The model under review builds one solid part; all positions refer to its coordinate system, in mm. A direction names the side the tool comes from. Round coordinates to 2 decimals unless told otherwise and drop trailing zeros. Write each loop counter-clockwise with the first axis right and the second up, starting at its lowest first coordinate (ties: lowest second). Pieces come first, ordered by that corner, then holes. Notation, with made-up numbers: (38, 14) -> (48, 14) arc R20 cw to (48, 43) -> close; hole circle Ø6 at (-17.75, 60.25). An arc over 180 degrees is marked (long way). Use CSV: the item, a comma, the result in double quotes. Start each with the question number.
1) Wall thickness on probe 1 along Y at (x, z) = (-0.4, 19.5); probe 2 along X at (y, z) = (-0.75, 12); probe 3 along Y at (x, z) = (10, 21): over which ranges is each line inside the solid? List them lowest first. Write a range as [from, to].
2) Machinability: for faces 4 (the face through (1, -7, 20)), 5 (the face through (4.5, 0, 20)), 6 (the face through (10.768, 7.436, 20.88)), which of the approach directions +Z, -Z, +X, -X, +Y, -Y give a long, thin tool a straight path to every point of the face, cutting with its end or side? Answer none if there is none.
3) Take a section at A-A, the plane x = -9.5. Give the boundary of the cut face in (y, z), then the cut area to 3 significant figures.
4) For pin 1 Ø6 at (y, z) = (-4, 5) entering from +X; pin 2 Ø7 at (y, z) = (5, 19.5) entering from +X; pin 3 Ø3 at (y, z) = (-4, 19.5) entering from +X; pin 4 Ø1.2 at (x, y) = (11, 4.5) entering from +Z, all flat-tipped, find the tip position at first contact; note any pin that passes through.
5) Take a section at B-B, the plane z = 12. Give the boundary of the cut face in (x, y), then the cut area to 3 significant figures.
6) Mouldability with a two-part tool opening along Z and no side actions: class faces 1 (the face through (14, 0, 3)), 2 (the face through (10.768, -7.436, 18.12)), 3 (the face through (-16.14, 9.1, 1.52)) as released by +Z, released by -Z, zero draft, split by the parting line, or undercut.
7) Take a section at C-C, the plane y = 0. Give the boundary of the cut face in (x, z), then the cut area to 3 significant figures.
8) Take a section at D-D, the plane y = 4. Give the boundary of the cut face in (x, z).
from build123d import *

# Parameters (mm, degrees)
SKETCH1_W           = 34
SKETCH1_H           = 20
BOSS_EXTRUDE1_DEPTH = 3
FILLET1_R           = 3
SKETCH2_W           = 14
SKETCH2_H           = 20
BOSS_EXTRUDE2_DEPTH = 20
CUT_EXTRUDE1_DEPTH  = 35.899856733
CHAMFER1_SIZE       = 1
SKETCH4_R           = 2.2
CUT_EXTRUDE2_DEPTH  = 29.08914381
SKETCH5_R           = 1.7
CUT_EXTRUDE3_DEPTH  = 39.340579025
FILLET2_R           = 2
CUT_EXTRUDE4_DEPTH  = 2.5
SKETCH7_R           = 2.75
CUT_EXTRUDE5_DEPTH  = 3


with BuildPart() as part:
    # Sketch1 → Boss-Extrude1 (new body)
    with BuildSketch(Plane.XY):
        Rectangle(SKETCH1_W, SKETCH1_H)
    extrude(amount=BOSS_EXTRUDE1_DEPTH)

    # Fillet1
    fillet1_edges = [part.edges().sort_by_distance(p)[0] for p in [
        (17, -10, 1.5),
        (-17, -10, 1.5),
        (-17, 10, 1.5),
        (17, 10, 1.5),
    ]]
    fillet(fillet1_edges, radius=FILLET1_R)

    # Sketch2 → Boss-Extrude2 (add)
    with BuildSketch(Plane.XY.offset(3)):
        with Locations((5, 0)):
            Rectangle(SKETCH2_W, SKETCH2_H)
    extrude(amount=BOSS_EXTRUDE2_DEPTH)

    # Sketch3 → Cut-Extrude1 (cut, through all)
    with BuildSketch(Plane(origin=(0, 10, 0), x_dir=(1, 0, 0), z_dir=(0, 1, 0))):
        with BuildLine():
            Line((4.5, -16.119769411), (4.5, -23))
            Line((4.5, -23), (5.5, -23))
            Line((5.5, -23), (5.5, -16.119769411))
            ThreePointArc((5.5, -16.119769411), (5, -7.85), (4.5, -16.119769411))
        make_face()
    extrude(amount=-CUT_EXTRUDE1_DEPTH, mode=Mode.SUBTRACT)

    # Chamfer1
    chamfer1_edges = [part.edges().sort_by_distance(p)[0] for p in [
        (5, -10, 7.85),
        (5, 10, 7.85),
    ]]
    chamfer(chamfer1_edges, length=CHAMFER1_SIZE)

    # Sketch4 → Cut-Extrude2 (cut, through all)
    with BuildSketch(Plane.XY.offset(3)):
        with Locations((-9.5, 0)):
            Circle(SKETCH4_R)
    extrude(amount=-CUT_EXTRUDE2_DEPTH, mode=Mode.SUBTRACT)

    # Sketch5 → Cut-Extrude3 (cut, through all)
    with BuildSketch(Plane(origin=(12, 0, 0), x_dir=(0, 0, -1), z_dir=(1, 0, 0))):
        with Locations(Location((-19.5, 5, 0), (0, 0, 90))):
            Circle(SKETCH5_R)
        with Locations(Location((-19.5, -5, 0), (0, 0, 90))):
            Circle(SKETCH5_R)
    extrude(amount=-CUT_EXTRUDE3_DEPTH, mode=Mode.SUBTRACT)

    # Fillet2
    # the kernel refuses this fillet: 2 mm, written as the material it takes off along each edge
    with BuildSketch(Plane(origin=(12, -15, 23), x_dir=(-1, 0, 0), z_dir=(0, 1, 0)), Plane(origin=(-2, 15, 23), x_dir=(1, 0, 0), z_dir=(0, -1, 0))) as fillet2_piece_1:
        with BuildLine():
            CenterArc((FILLET2_R, -FILLET2_R), FILLET2_R, 90, 90)
            Line((0, -FILLET2_R), (0, 0))
            Line((0, 0), (FILLET2_R, 0))
        make_face()
    extrude(amount=30, mode=Mode.SUBTRACT)

    # Sketch6 → Cut-Extrude4 (cut)
    with BuildSketch(Plane(origin=(12, 0, 0), x_dir=(0, 0, -1), z_dir=(1, 0, 0))):
        Polygon((-16.7, 3.383419246), (-16.7, 6.616580754), (-19.5, 8.233161507), (-22.3, 6.616580754), (-22.3, 3.383419246), (-19.5, 1.766838493), align=None)
        Polygon((-16.7, -3.383419246), (-19.5, -1.766838493), (-22.3, -3.383419246), (-22.3, -6.616580754), (-19.5, -8.233161507), (-16.7, -6.616580754), align=None)
    extrude(amount=-CUT_EXTRUDE4_DEPTH, mode=Mode.SUBTRACT)

    # Sketch7 → Cut-Extrude5 (cut)
    with BuildSketch(Plane.ZY.offset(2)):
        with Locations(Location((19.5, 5, 0), (0, 0, 270))):
            Circle(SKETCH7_R)
        with Locations(Location((19.5, -5, 0), (0, 0, 270))):
            Circle(SKETCH7_R)
    extrude(amount=-CUT_EXTRUDE5_DEPTH, mode=Mode.SUBTRACT)


solid = part.part
Values found:
1,probe 1,"[-10, -7.75], [-2.25, 2.25], [7.75, 10]"
1,probe 2,"[-2, 0.85], [9.15, 12]"
1,probe 3,"[-10, -7.37], [-2.63, 2.63], [7.37, 10]"
2,face 4,"-X"
2,face 5,"+Z, +Y, -Y"
2,face 6,"+X"
3,outline,"(-10, 0) -> (-2.2, 0) -> (-2.2, 3) -> (-10, 3) -> close; (2.2, 0) -> (10, 0) -> (10, 3) -> (2.2, 3) -> close"
3,area,"46.8 mm²"
4,pin 1,"x = 17"
4,pin 2,"x = 12"
4,pin 3,"x = 9.5"
4,pin 4,"z = 22.96"
5,outline,"(-2, -10) -> (-0.15, -10) -> (0.85, -9) -> (0.85, 9) -> (-0.15, 10) -> (-2, 10) -> close; (9.15, -9) -> (10.15, -10) -> (12, -10) -> (12, 10) -> (10.15, 10) -> (9.15, 9) -> close"
5,area,"112 mm²"
6,face 1,"released by +Z"
6,face 2,"undercut"
6,face 3,"zero draft"
7,outline,"(-17, 0) -> (-11.7, 0) -> (-11.7, 3) -> (-17, 3) -> close; (-7.3, 0) -> (17, 0) -> (17, 3) -> (12, 3) -> (12, 21) arc R2 ccw to (10, 23) -> (5.5, 23) -> (5.5, 16.12) arc R4.15 cw (long way) to (4.5, 16.12) -> (4.5, 23) -> (0, 23) arc R2 ccw to (-2, 21) -> (-2, 3) -> (-7.3, 3) -> close"
7,area,"306 mm²"
8,outline,"(-17, 0) -> (17, 0) -> (17, 3) -> (12, 3) -> (12, 16.7) -> (9.5, 16.7) -> (9.5, 18.13) -> (5.5, 18.13) -> (5.5, 16.12) arc R4.15 cw (long way) to (4.5, 16.12) -> (4.5, 18.13) -> (1, 18.13) -> (1, 16.94) -> (-2, 16.94) -> (-2, 3) -> (-17, 3) -> close; (-1.69, 22.06) -> (1, 22.06) -> (1, 20.87) -> (4.5, 20.87) -> (4.5, 23) -> (0, 23) arc R2 ccw to start; (5.5, 20.87) -> (9.5, 20.87) -> (9.5, 22.3) -> (11.52, 22.3) arc R2 ccw to (10, 23) -> (5.5, 23) -> close"
